Read the model definition and answer for the solid it produces. Units are mm, in the model's axes. Face numbers are marked on the shaded views. A direction names the side the tool comes from. Coordinates: 2 decimals unless noted, no trailing zeros. Order: outer loops, then holes, each group sorted by start corner. A loop starts at its lowest first (then second) coordinate and runs counter-clockwise, first axis right, second up. Notation, with made-up numbers: M -1.75,87.25 L 48.25,87.25 A31 ccw 48.25,118.25 Z; hole C 40,75 d4. An arc over 180 degrees is marked long. Write each question's results on one line, items separated by ' | '.
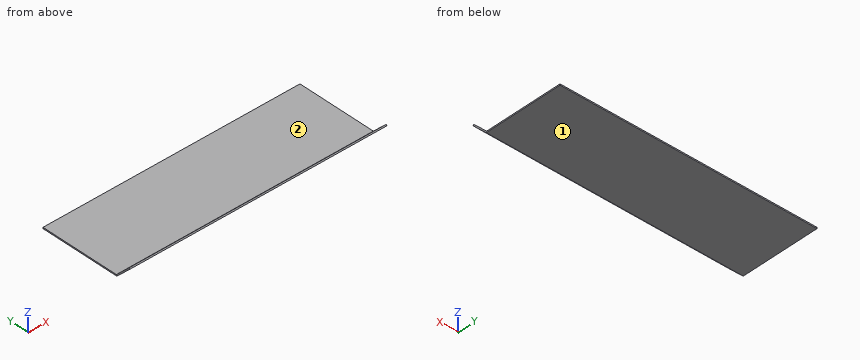
Autodesk Inventor part; units mm, degrees
ref_plane "YZ Plane" through (0, 0, 0) normal (1, 0, 0) x (0, 1, 0)
ref_plane "XZ Plane" through (0, 0, 0) normal (0, 1, 0) x (-1, 0, 0)
ref_plane "XY Plane" through (0, 0, 0) normal (0, 0, 1) x (1, 0, 0)
sketch "Sketch1" plane through (0, 0, 0) normal (1, 0, 0) x (0, 1, 0)
  line L0 (0, 0) -> (101.6, 0)
  line L1 (101.6, 0) -> (101.6, -1.5875)
  line L2 (101.6, -1.5875) -> (0, -1.5875)
  line L3 (0, -1.5875) -> (0, 0)
  circle A0 centre (0, -0.7937) radius 0.7937
  line L4 (0.5613, -0.2325) -> (-17.3992, 17.728)
  line L5 (-0.5613, -1.355) -> (-18.5218, 16.6055)
  line L6 (-17.3992, 17.728) -> (-18.5218, 16.6055)
  point P0 (0.3288, 0)
  dimension "d0" = 101.6
  dimension "d1" = 1.5875
  dimension "d2" = 25.4
  dimension "d3" = 135
  dimension "d4" = 25.4
extrude "Extrusion1" add sketch "Sketch1" along normal blind 330.2
properties part number "Wedge" material "Polycarbonate, Clear"
(1) Given pin 1 (10 mm diameter, centred on x = 162.5, z = 9.5, fed in from +Y); pin 2 (12 mm diameter, centred on x = 292, y = 32.5, fed in from +Z); pin 3 (6 mm diameter, centred on x = 261.5, z = 3.5, fed in from -Y), each flat-ended and moving along its own axis, determine where each tip first touches the part or whether it passes through.
Conclusion:
pin 1: y = -4.17 | pin 2: z = 0 | pin 3: y = -8.42
(2) For the marked faces 1 and 2, determine the directions among +Z, -Z, +X, -X, +Y, -Y from which every point of the face is accessible in a straight line to the end or side of a thin tool.
Conclusion:
face 1: -Z, +X, -X, +Y, -Y | face 2: +Z, +X, -X, +Y
(3) The part is cut by section C-C, the plane z = 10.25. Write down the section's boundary in (x, y).
Conclusion:
outline: M 0,-12.17 L 330.2,-12.17 L 330.2,-9.92 L 0,-9.92 Z
(4) The part is cut by section B-B, the plane x = 61.5. Write down the section's boundary in (y, z) (1 decimal).
Conclusion:
outline: M -18.5,16.6 L -0.6,-1.4 A0.8 ccw 0,-1.6 L 101.6,-1.6 L 101.6,0 L 0.3,0 L -17.4,17.7 Z
(5) Straight lines are drawn through the part: line 1 (Z direction, x = 284.5, y = 44); line 2 (Y direction, x = 297, z = 13); line 3 (Z direction, x = 222, y = -2.5). For each, find the intervals that lie inside material, in ascending order.
Conclusion:
line 1: -1.59 to 0 | line 2: -14.92 to -12.67 | line 3: 0.58 to 2.83
(6) The part is cut by section A-A, the plane y = 81. Write down the section's boundary in (x, z).
Conclusion:
outline: M 0,-1.59 L 330.2,-1.59 L 330.2,0 L 0,0 Z
